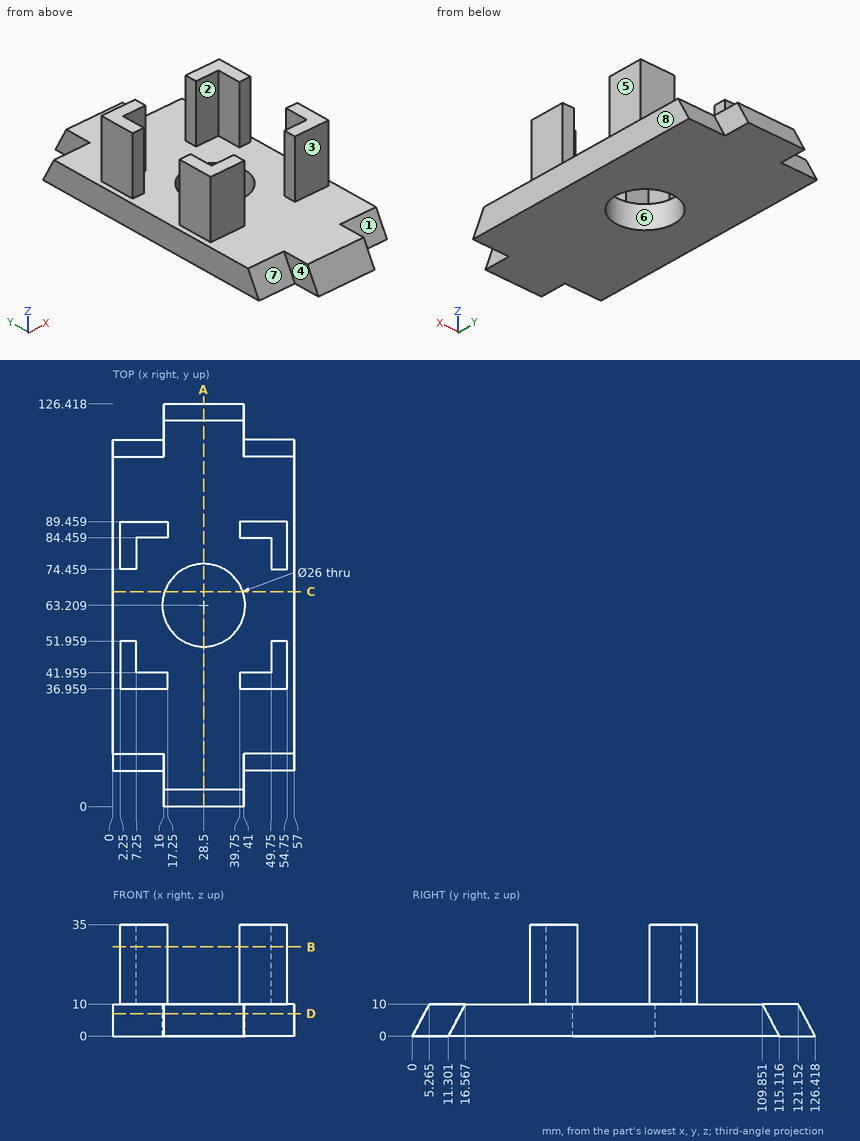
Job drawing, mm, ordinate dimensions from the low corner. One solid piece. A direction names the side the tool comes from. Coordinates: 2 decimals unless noted, no trailing zeros. Order: outer loops, then holes, each group sorted by start corner. A loop starts at its lowest first (then second) coordinate and runs counter-clockwise, first axis right, second up. Notation, with made-up numbers: (59.5, 3.25) -> (84.5, 3.25) arc R19 cw to (84.5, 14.25) -> close; hole circle Ø7 at (-19.5, 89). An arc over 180 degrees is marked (long way). Return JSON: item names as keys, results as strings. Group by question number.
Item 1: Saw through at D-D on z = 7. Write the cut outline in (x, y) (1 decimal).
Item 2: Saw through at A-A on x = 28.5. Write the cut outline in (y, z) (1 decimal).
Item 3: Saw through at C-C on y = 67.5. Write the cut outline in (x, z).
Item 4: Wall check: line 1 along Y through (x, z) = (47, 10.5); line 2 along X through (y, z) = (44, 19.5); line 3 along Z through (x, y) = (27, 6.5). Give the ranges that are in metal, low to high. Write a range as [from, to].
Item 5: Flat gauge pins, fed straight in: P1, Ø12, axis at x = 49, z = 8.5, coming from the -Y side; P2, Ø12, axis at x = 49.5, z = 17, coming from the -Y side; P3, Ø2.5, axis at x = 52.5, z = 19.5, coming from the +Y side; P4, Ø12, axis at y = 96.5, z = 19.5, coming from the +X side. Where does each tip first touch, or does it go through?
Item 6: Pull direction X, two halves, no side cores. Call the marked faces 6, 7 and 8: pulls with the +X half, pulls with the -X half, needs draft (parallel to the pull), parting line crosses it, or undercut.
Item 7: Saw through at B-B on z = 28. Write the cut outline in (x, y), then the cut area to 3 significant figures.
Item 8: Tool access for the marked faces 1, 2, 3, 4 and 5: list every direction of +Z, -Z, +X, -X, +Y, -Y with a clear straight run to the whole face (end or side of a thin tool).
Values found:
{
 "1": {"outline": "(0, 15) -> (16, 15) -> (16, 3.7) -> (41, 3.7) -> (41, 15) -> (57, 15) -> (57, 111.4) -> (41, 111.4) -> (41, 122.7) -> (16, 122.7) -> (16, 111.4) -> (0, 111.4) -> close; hole circle Ø26 at (28.5, 63.2)"},
 "2": {"outline": "(0, 0) -> (50.2, 0) -> (50.2, 10) -> (5.3, 10) -> close; (76.2, 0) -> (126.4, 0) -> (121.2, 10) -> (76.2, 10) -> close"},
 "3": {"outline": "(0, 0) -> (16.23, 0) -> (16.23, 10) -> (0, 10) -> close; (40.77, 0) -> (57, 0) -> (57, 10) -> (40.77, 10) -> close"},
 "4": {"line 1": "y = [36.96, 41.96], [84.46, 89.46]", "line 2": "x = [2.25, 7.25], [49.75, 54.75]", "line 3": "z = [0, 10]"},
 "5": {"P1": "stops at y = 12.62", "P2": "stops at y = 36.96", "P3": "stops at y = 89.46", "P4": "passes through"},
 "6": {"face 6": "undercut", "face 7": "needs draft", "face 8": "pulls with the +X half"},
 "7": {"outline": "(2.25, 36.96) -> (17.25, 36.96) -> (17.25, 41.96) -> (7.25, 41.96) -> (7.25, 51.96) -> (2.25, 51.96) -> close; (2.25, 74.46) -> (7.25, 74.46) -> (7.25, 84.46) -> (17.25, 84.46) -> (17.25, 89.46) -> (2.25, 89.46) -> close; (39.75, 36.96) -> (54.75, 36.96) -> (54.75, 51.96) -> (49.75, 51.96) -> (49.75, 41.96) -> (39.75, 41.96) -> close; (39.75, 84.46) -> (49.75, 84.46) -> (49.75, 74.46) -> (54.75, 74.46) -> (54.75, 89.46) -> (39.75, 89.46) -> close", "area": "500 mm2"},
 "8": {"face 1": "+Z, +X, -Y", "face 2": "+Z", "face 3": "+Z, +X, -X, -Y", "face 4": "+Z, -X, -Y", "face 5": "+Z, +X, +Y, -Y"}
}
